```python
from build123d import *

# Parameters (mm, degrees)
F0_R     = 12.7
F1_DEPTH = 6.35


with BuildPart() as f1:
    # F0 (on Top) → F1 (new body)
    with BuildSketch(Plane.XY):
        with BuildLine():
            Line((0, -8.536373), (0, 41.326012))
            Line((0, 41.326012), (-95.25, 41.326012))
            ThreePointArc((-95.25, 41.326012), (-100.672652, 38.280153), (-100.893214, 32.064546))
            Line((-100.893214, 32.064546), (-65.33969, -36.84784))
            ThreePointArc((-65.33969, -36.84784), (-63.000616, -39.359026), (-59.696476, -40.286373))
            Line((-59.696476, -40.286373), (0, -40.286373))
            Line((0, -40.286373), (0, -33.936373))
            ThreePointArc((0, -33.936373), (-12.7, -21.236373), (0, -8.536373))
        make_face()
        with Locations((-73.025, 21.980401)):
            Circle(F0_R, mode=Mode.SUBTRACT)
        with BuildLine():
            Line((95.25, 41.326012), (0, 41.326012))
            Line((0, 41.326012), (0, -8.536373))
            ThreePointArc((0, -8.536373), (12.7, -21.236373), (0, -33.936373))
            Line((0, -33.936373), (0, -40.286373))
            Line((0, -40.286373), (59.696476, -40.286373))
            ThreePointArc((59.696476, -40.286373), (63.000616, -39.359026), (65.33969, -36.84784))
            Line((65.33969, -36.84784), (100.893214, 32.064546))
            ThreePointArc((100.893214, 32.064546), (100.672652, 38.280153), (95.25, 41.326012))
        make_face()
        with Locations((73.025, 21.980401)):
            Circle(F0_R, mode=Mode.SUBTRACT)
    extrude(amount=F1_DEPTH)


solid = f1.part
```
Verification items for the finished model (mm, model axes). Coordinates: 2 decimals unless noted, no trailing zeros. Order: outer loops, then holes, each group sorted by start corner. A loop starts at its lowest first (then second) coordinate and runs counter-clockwise, first axis right, second up. Notation, with made-up numbers: (85.25, 18.5) -> (103.25, 18.5) arc R16 cw to (103.25, 34.5) -> close; hole circle Ø1 at (72, 11.25). An arc over 180 degrees is marked (long way). Put each result on its own line as item: value. Start each with the question number.
1) Cross-section at C-C (y = -29.5). Enter the section's corners in (x, z).
2) Material ranges on L1, parallel to X at y = 19.5, z = 2.25; L2, parallel to X at y = -24.5, z = 2; L3, parallel to Y at x = 66.5, z = 4, recorded low to high.
3) Release check for a two-part mould opening along Y. For faces 1 (the flat face through (-1, 1, 0)), 2 (the cylindrical face through (-100.6, 38.4, 3.1)), 3 (the cylindrical face through (-63.042, -39.334, 3.131)), 4 (the cylindrical face through (-60.911, 25.795, 3.131)) record: pulls with the +Y half, pulls with the -Y half, needs draft (parallel to the pull), parting line crosses it, or undercut.
4) Cross-section at B-B (y = 27.5). Enter the section's corners in (x, z).
5) Cross-section at A-A (x = 0). Enter the section's corners in (y, z).
6) Cross-section at D-D (z = 3.5). Enter the section's corners in (x, y) (3 decimals), plus the area to 3 significant figures.
7) Go/stop test with flat-tipped pins: pin 1 (2 mm diameter, centred on y = 3, z = 4.5, fed in from +X); pin 2 (1.5 mm diameter, centred on y = 28.5, z = 1.5, fed in from +X); pin 3 (23 mm diameter, centred on x = 0, y = -21.24, fed in from +Z). Record where each tip stops, or that it passes through.
Geometry check:
1. outline: (-69.13, 0) -> (-9.64, 0) -> (-9.64, 6.35) -> (-69.13, 6.35) -> close; (9.64, 0) -> (69.13, 0) -> (69.13, 6.35) -> (9.64, 6.35) -> close
2. L1: x = -94.41 to -85.48, -60.57 to 60.57, 85.48 to 94.41
2. L2: x = -71.71 to -12.27, 12.27 to 71.71
2. L3: y = -34.6 to 11.08, 32.88 to 41.33
3. face 1: needs draft
3. face 2: parting line crosses it
3. face 3: pulls with the -Y half
3. face 4: undercut
4. outline: (-98.54, 0) -> (-84.46, 0) -> (-84.46, 6.35) -> (-98.54, 6.35) -> close; (-61.59, 0) -> (61.59, 0) -> (61.59, 6.35) -> (-61.59, 6.35) -> close; (84.46, 0) -> (98.54, 0) -> (98.54, 6.35) -> (84.46, 6.35) -> close
5. outline: (-40.29, 0) -> (-33.94, 0) -> (-33.94, 6.35) -> (-40.29, 6.35) -> close; (-8.54, 0) -> (41.33, 0) -> (41.33, 6.35) -> (-8.54, 6.35) -> close
6. outline: (-100.893, 32.065) -> (-65.34, -36.848) arc R6.35 ccw to (-59.696, -40.286) -> (59.696, -40.286) arc R6.35 ccw to (65.34, -36.848) -> (100.893, 32.065) arc R6.35 ccw to (95.25, 41.326) -> (-95.25, 41.326) arc R6.35 ccw to start; hole circle Ø25.4 at (-73.025, 21.98); hole circle Ø25.4 at (0, -21.236); hole circle Ø25.4 at (73.025, 21.98)
6. area: 12,200 mm^2
7. pin 1: stops at x = 86.41
7. pin 2: stops at x = 99.44
7. pin 3: passes through
